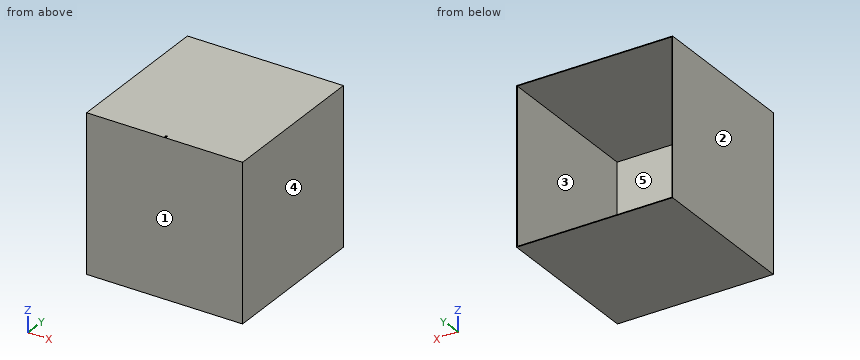
Autodesk Fusion 360 part; units mm, degrees
sketch "Sketch1" plane through (0, 0, 0) normal (0, 1, 0) x (1, 0, 0)
  line L0 (300, -300) -> (-300, -300)
  line L1 (-300, -300) -> (-300, 300)
  line L2 (-300, 300) -> (300, 300)
  line L3 (300, 300) -> (300, -300)
  line L4 (300, -300) -> (-300, 300) construction
  line L5 (-300, -300) -> (300, 300) construction
  dimension "d1" = 600
  dimension "d2" = 600
extrude "Extrude1" add sketch "Sketch1" along normal blind 600 in component "Component"
sketch "Sketch2" plane through (0, 600, 0) normal (0, 1, 0) x (-1, 0, 0)
  line L0 (-300, -300) -> (300, -300)
  line L1 (300, -300) -> (300, 300)
  line L2 (300, 300) -> (-300, 300)
  line L3 (-300, 300) -> (-300, -300)
  line L4 (-297.5, 297.5) -> (297.5, 297.5)
  line L5 (297.5, 297.5) -> (297.5, -297.5)
  line L6 (297.5, -297.5) -> (-297.5, -297.5)
  line L7 (-297.5, -297.5) -> (-297.5, 297.5)
  line L8 (-297.5, 297.5) -> (297.5, -297.5) construction
  line L9 (297.5, 297.5) -> (-297.5, -297.5) construction
  dimension "d5" = 595
  dimension "d6" = 595
extrude "Extrude2" cut sketch "Sketch2" against normal blind 595 contours L4 L5 L6 L7 in component "Component"
sketch "Sketch3" plane through (0, 0, 300) normal (0, 0, 1) x (1, 0, 0)
  line L0 (-300, 0) -> (300, 0)
  line L1 (300, 0) -> (300, 600)
  line L2 (300, 600) -> (-300, 600)
  line L3 (-300, 600) -> (-300, 0)
  circle A0 centre (0, 9) radius 4
  point P0 (0, 5)
  point P1 (0, 9)
  dimension "d9" = 5
  dimension "d10" = 4
  dimension "d11" = 8
extrude "Extrude3" cut sketch "Sketch3" against normal blind 30 contours A0 in component "Component"
component "Component" placed x (1, 0, 0) y (0, 1, 0) z (0, 0, 1) at (0, 0, 0)
Could you check a few things on this model? Use its own coordinates, in mm. Face numbers are marked on the shaded views. A direction names the side the tool comes from. Coordinates: 2 decimals unless noted, no trailing zeros. Loops run counter-clockwise (first coordinate to the right, second up) from the corner with the lowest first, then second, coordinate; pieces in that order, holes last.
1. We'd pull the mould along X, two halves only. Please class the marked faces 1, 2 and 3: released by +X, released by -X, zero draft, split by the parting line, or undercut.
2. I need wall thicknesses on L1, parallel to X at y = 506.5, z = 206.5; L2, parallel to X at y = 9, z = 299. Which ranges of each line are inside material? Lowest first, please.
3. Imagine slicing it at A-A (y = 483). Please give me the cut outline in (x, z).
4. Imagine slicing it at B-B (x = -51). Please give me the cut outline in (y, z), and give its area (4 significant figures).
5. For the marked faces 4 and 5, which set-ups out of +Z, -Z, +X, -X, +Y, -Y let a thin tool reach every point of the face, with its end or its side?
6. Imagine slicing it at C-C (z = 155.5). Please give me the cut outline in (x, y), and give its area (4 significant figures).
Computed values:
1. face 1: zero draft
1. face 2: released by -X
1. face 3: undercut
2. L1: x = -300 to -297.5, 297.5 to 300
2. L2: x = -300 to -4, 4 to 300
3. outline: (-300, -300) - (300, -300) - (300, 300) - (-300, 300) - close; hole (-297.5, -297.5) - (297.5, -297.5) - (297.5, 297.5) - (-297.5, 297.5) - close
4. outline: (0, -300) - (600, -300) - (600, -297.5) - (5, -297.5) - (5, 297.5) - (600, 297.5) - (600, 300) - (0, 300) - close
4. area: 5,975 mm2
5. face 4: +Z, -Z, +X, +Y, -Y
5. face 5: +Y
6. outline: (-300, 0) - (300, 0) - (300, 600) - (297.5, 600) - (297.5, 5) - (-297.5, 5) - (-297.5, 600) - (-300, 600) - close
6. area: 5,975 mm2
